Could you check a few things on this drawing? It's one solid part, dimensions in mm from its lowest x, y, z. A direction names the side the tool comes from. Round coordinates to 2 decimals unless told otherwise and drop trailing zeros. Write each loop counter-clockwise with the first axis right and the second up, starting at its lowest first coordinate (ties: lowest second). Pieces come first, ordered by that corner, then holes. Notation, with made-up numbers: (29, 82) -> (69, 82) arc R10 cw to (69, 89) -> close; hole circle Ø1 at (84, 33.25). An arc over 180 degrees is marked (long way). Answer as CSV lines item,"result".
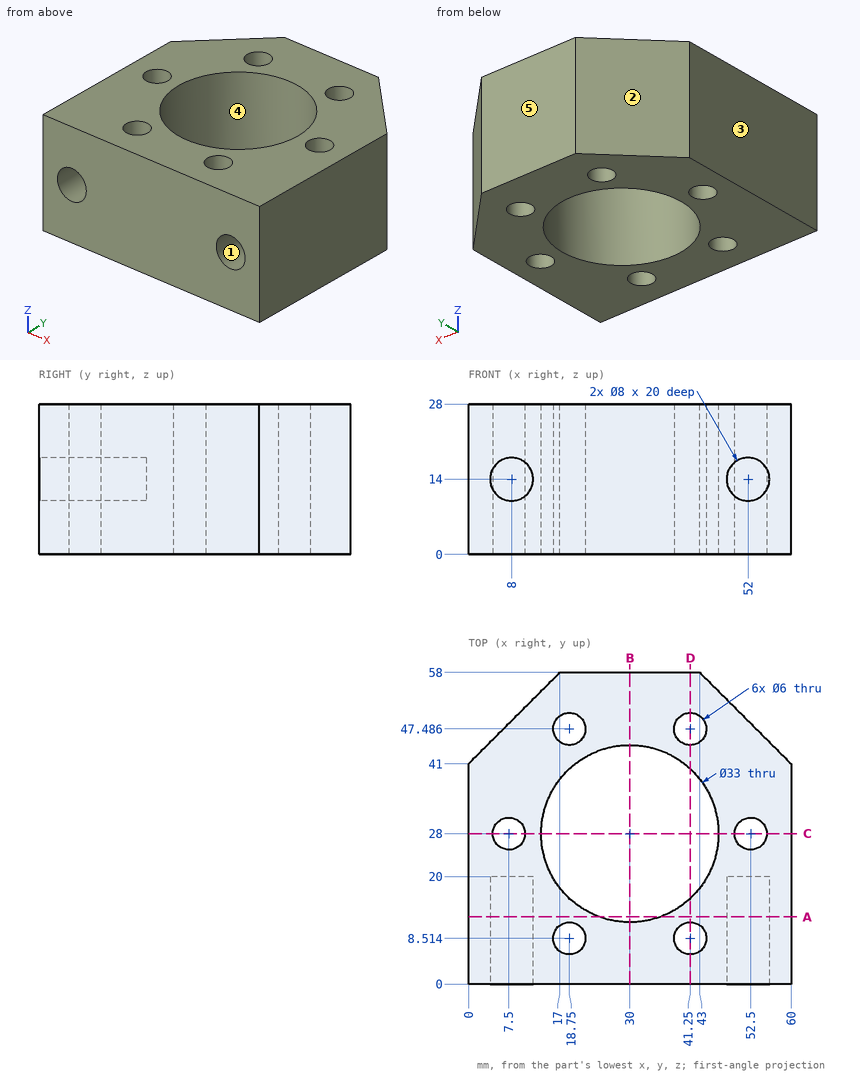
1. Suppose I cut it at A-A on y = 12.5. Please give me the cut outline in (x, z).
Numbers:
outline,"(0, 0) -> (24.34, 0) -> (24.34, 28) -> (0, 28) -> close; (35.66, 0) -> (60, 0) -> (60, 28) -> (35.66, 28) -> close; hole circle Ø8 at (8, 14); hole circle Ø8 at (52, 14)"
2. If we mould it in two halves opening along X, with no side actions, what happens to the marked faces 3, 4 and 5? For each: released by +X, released by -X, zero draft, split by the parting line, or undercut.
Numbers:
face 3,"released by -X"
face 4,"undercut"
face 5,"zero draft"
3. On a 3-axis mill with a long thin cutter (end or side, diameter ignored), from which of +Z, -Z, +X, -X, +Y, -Y can I reach the whole of each face in a straight line? I mean the marked faces 1 and 2. Say none if no direction works.
Numbers:
face 1,"-Y"
face 2,"+Z, -Z, -X, +Y"
4. Suppose I cut it at D-D on x = 41.25. Please give me the cut outline in (y, z) (1 decimal).
Numbers:
outline,"(0, 0) -> (5.5, 0) -> (5.5, 28) -> (0, 28) -> close; (11.5, 0) -> (15.9, 0) -> (15.9, 28) -> (11.5, 28) -> close; (40.1, 0) -> (44.5, 0) -> (44.5, 28) -> (40.1, 28) -> close; (50.5, 0) -> (58, 0) -> (58, 28) -> (50.5, 28) -> close"
5. For pin 1 Ø7 at (x, y) = (7.5, 28) entering from +Z; pin 2 Ø2.5 at (x, z) = (6, 15) entering from -Y; pin 3 Ø12 at (x, z) = (52, 13) entering from +Y; pin 4 Ø5 at (x, z) = (52, 14) entering from +Y, each with a flat end and sliding along its axis, tell me the tip position at first contact or that it passes through.
Numbers:
pin 1,"stops at z = 28"
pin 2,"stops at y = 20"
pin 3,"stops at y = 55"
pin 4,"stops at y = 51.5"
6. If I drill on line 1 (Y direction, x = 39, z = 4.5); line 2 (Y direction, x = 40.5, z = 3.75); line 3 (Y direction, x = 29, z = 23.5), over which ranges is the centre line in solid material (lowest first)?
Numbers:
line 1,"y = 0 to 6.53, 10.5 to 14.17, 41.83 to 45.5, 49.47 to 58"
line 2,"y = 0 to 5.61, 11.42 to 15.27, 40.73 to 44.58, 50.39 to 58"
line 3,"y = 0 to 11.53, 44.47 to 58"
7. Suppose I cut it at C-C on y = 28. Please give me the cut outline in (x, z).
Numbers:
outline,"(0, 0) -> (4.5, 0) -> (4.5, 28) -> (0, 28) -> close; (10.5, 0) -> (13.5, 0) -> (13.5, 28) -> (10.5, 28) -> close; (46.5, 0) -> (49.5, 0) -> (49.5, 28) -> (46.5, 28) -> close; (55.5, 0) -> (60, 0) -> (60, 28) -> (55.5, 28) -> close"
8. Suppose I cut it at B-B on x = 30. Please give me the cut outline in (y, z).
Numbers:
outline,"(0, 0) -> (11.5, 0) -> (11.5, 28) -> (0, 28) -> close; (44.5, 0) -> (58, 0) -> (58, 28) -> (44.5, 28) -> close"
